The model under review builds one solid part; all positions refer to its coordinate system, in mm. Round coordinates to 2 decimals unless told otherwise and drop trailing zeros. Write each loop counter-clockwise with the first axis right and the second up, starting at its lowest first coordinate (ties: lowest second). Pieces come first, ordered by that corner, then holes. Notation, with made-up numbers: (15, 45) -> (61, 45) arc R13 cw to (61, 61) -> close; hole circle Ø11 at (-40, 75). An arc over 180 degrees is marked (long way). Use CSV: the item, a comma, the result in double quotes. Start each with the question number.
1) Take a section at A-A, the plane z = 13. Give the boundary of the cut face in (x, y).
2) For pin 1 Ø4 at (y, z) = (20.5, 8) entering from +X; pin 2 Ø4 at (x, z) = (-33.5, 5) entering from +Y; pin 3 Ø2 at (x, z) = (-2.5, 11) entering from +Y, all flat-tipped, find the tip position at first contact; note any pin that passes through.
3) Wall thickness on probe 1 along Y at (x, z) = (2, 2.75); probe 2 along Z at (x, y) = (1.5, -11); probe 3 along Z at (x, y) = (-36, 3.5): over which ranges is each line inside the solid? List them lowest first. Write a range as [from, to].
4) Take a section at B-B, the plane z = 6.25. Give the boundary of the cut face in (x, y), then the cut area to 3 significant figures.
from build123d import *

# Parameters (mm, degrees)
F0_R     = 25
F1_DEPTH = 17
F2_SIZE  = 15


# Not quite as in the source:
# - a fillet or chamfer that OpenCascade refuses, or shapes differently, is made with other operations: its cross-section is extruded or revolved along the edge and cut away or added


with BuildPart() as f1:
    # F0 (on Top) → F1 (new body)
    with BuildSketch(Plane.XY):
        with Locations((-14.6842114627, 6.9868424907)):
            Circle(F0_R)
    extrude(amount=F1_DEPTH)

    # F2
    f2_edges = [f1.edges().sort_by_distance(p)[0] for p in [
        (-39.684211, 6.986842, 17),
    ]]
    chamfer(f2_edges, length=F2_SIZE)

    # F3: fillet of radius 5 on 1 edges, made by hand

    # F3_s1 → F3_t2 (revolve, cut)
    with BuildSketch(Plane.XZ.offset(-6.9868424907)):
        with BuildLine():
            ThreePointArc((10.3157885373, 2), (8.5518565148, 0.527864045), (6.3157885373, 0))
            Line((6.3157885373, 0), (10.3157885373, 0))
            Line((10.3157885373, 0), (10.3157885373, 2))
        make_face()
    revolve(axis=Axis((-14.6842114627, 6.9868424907, 0), (0, 0, 1)), mode=Mode.SUBTRACT)


solid = f1.part
Values found:
1,outline,"circle Ø28 at (-14.68, 6.99)"
2,pin 1,"x = 1.85"
2,pin 2,"y = 22.69"
2,pin 3,"y = 19.16"
3,probe 1,"[-10.61, 24.59]"
3,probe 2,"[1.15, 2.8]"
3,probe 3,"[0.04, 5.4]"
4,outline,"circle Ø41.5 at (-14.68, 6.99)"
4,area,"1,350 mm²"
